The figure shows three views and two pictorial views of one solid part (mm, origin at its lowest corner). Answer the questions. Round coordinates to 2 decimals unless told otherwise and drop trailing zeros. Order: outer loops, then holes, each group sorted by start corner. A loop starts at its lowest first (then second) coordinate and runs counter-clockwise, first axis right, second up. Notation, with made-up numbers: (32, -6) - (41, -6) arc R16 cw to (41, 3) - close; hole circle Ø4 at (89, 17.5). An arc over 180 degrees is marked (long way). Use CSV: the item, a comma, the result in double quotes. Start each with the question number.
Item 1: Find section D-D, the plane y = 0.55. Count the separate pieces of the cut face and the enclosed holes in it, plus the area to 3 significant figures.
Item 2: Find section B-B, the plane x = 60. Give the vertices of the cut face in (y, z).
Item 3: Straight lines are drawn through the part: line 1 along X through (y, z) = (1.8, 20); line 2 along X through (y, z) = (0.8, 6); line 3 along Z through (x, y) = (74, 1.55). For each, find the intervals that lie inside material, in ascending order. Write a range as [from, to].
Item 4: Find section C-C, the plane x = 47.5. Give the vertices of the cut face in (y, z), plus the area to 3 significant figures.
Item 5: Find section A-A, the plane z = 20. Give the vertices of the cut face in (x, y).
Item 6: A flat-ended cylindrical pin translates along its axis: P1, Ø6, axis at x = 20, z = 20, coming from the -Y side. Find the tip coordinate at first contact, or state that the pin passes through.
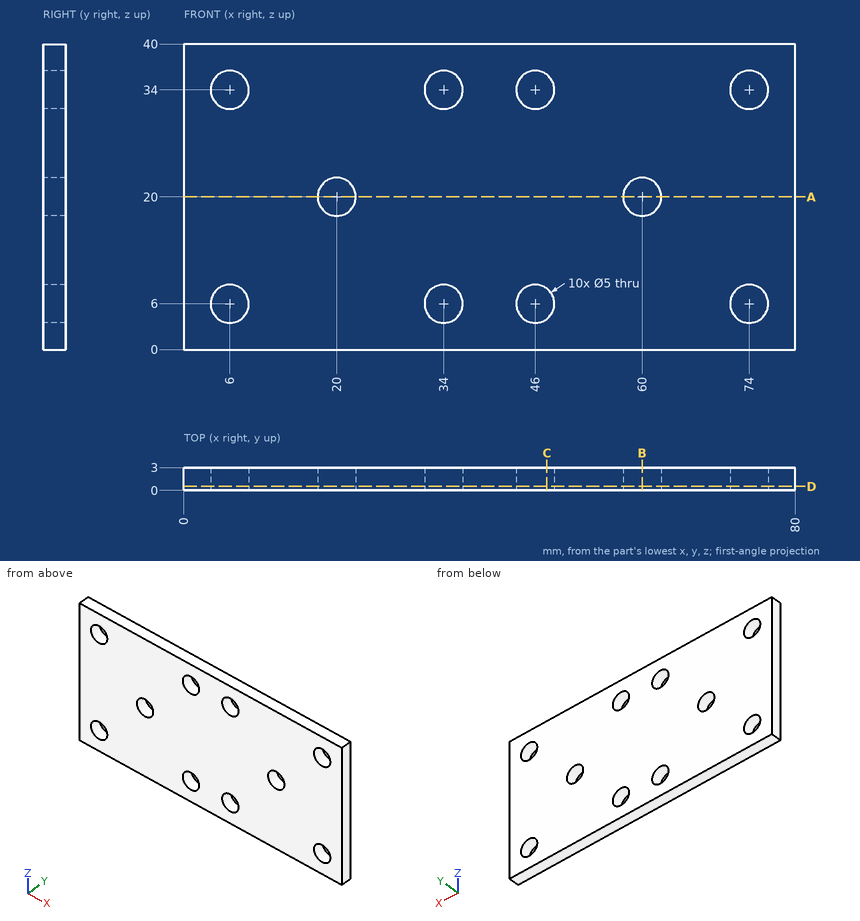
Worked out:
1,separate pieces,"1"
1,enclosed holes,"10"
1,area,"3,000 mm²"
2,outline,"(0, 0) - (3, 0) - (3, 17.5) - (0, 17.5) - close; (0, 22.5) - (3, 22.5) - (3, 40) - (0, 40) - close"
3,line 1,"x = [0, 17.5], [22.5, 57.5], [62.5, 80]"
3,line 2,"x = [0, 3.5], [8.5, 31.5], [36.5, 43.5], [48.5, 71.5], [76.5, 80]"
3,line 3,"z = [0, 3.5], [8.5, 31.5], [36.5, 40]"
4,outline,"(0, 0) - (3, 0) - (3, 4) - (0, 4) - close; (0, 8) - (3, 8) - (3, 32) - (0, 32) - close; (0, 36) - (3, 36) - (3, 40) - (0, 40) - close"
4,area,"96.0 mm²"
5,outline,"(0, 0) - (17.5, 0) - (17.5, 3) - (0, 3) - close; (22.5, 0) - (57.5, 0) - (57.5, 3) - (22.5, 3) - close; (62.5, 0) - (80, 0) - (80, 3) - (62.5, 3) - close"
6,P1,"stops at y = 0"
